from build123d import *

# Parameters (mm, degrees)
SKETCH2_R           = 2.5
BOSS_EXTRUDE1_DEPTH = 3


with BuildPart() as part:
    # Sketch2 → Boss-Extrude1 (new body)
    with BuildSketch(Plane(origin=(0, 0, 0), x_dir=(1, 0, 0), z_dir=(0, 1, 0))):
        with BuildLine():
            Line((-43.63, 60), (43.63, 60))
            ThreePointArc((43.63, 60), (46.896833329, 58.646833329), (48.25, 55.38))
            Line((48.25, 55.38), (48.25, 4.62))
            ThreePointArc((48.25, 4.62), (46.896833329, 1.353166671), (43.63, 0))
            Line((43.63, 0), (-43.63, 0))
            ThreePointArc((-43.63, 0), (-46.896833329, 1.353166671), (-48.25, 4.62))
            Line((-48.25, 4.62), (-48.25, 55.38))
            ThreePointArc((-48.25, 55.38), (-46.896833329, 58.646833329), (-43.63, 60))
        make_face()
        with Locations((-42.13, 6.43)):
            Circle(SKETCH2_R, mode=Mode.SUBTRACT)
        with Locations((-42.13, 53.57)):
            Circle(SKETCH2_R, mode=Mode.SUBTRACT)
        with Locations((5.01, 53.57)):
            Circle(SKETCH2_R, mode=Mode.SUBTRACT)
        with Locations((5.01, 6.43)):
            Circle(SKETCH2_R, mode=Mode.SUBTRACT)
        with BuildLine():
            Line((18.61, 52.5), (40.21, 52.5))
            ThreePointArc((40.21, 52.5), (42.71, 50), (40.21, 47.5))
            Line((40.21, 47.5), (18.61, 47.5))
            ThreePointArc((18.61, 47.5), (16.11, 50), (18.61, 52.5))
        make_face(mode=Mode.SUBTRACT)
        with BuildLine():
            Line((18.61, 7.5), (40.21, 7.5))
            ThreePointArc((40.21, 7.5), (42.71, 10), (40.21, 12.5))
            Line((40.21, 12.5), (18.61, 12.5))
            ThreePointArc((18.61, 12.5), (16.11, 10), (18.61, 7.5))
        make_face(mode=Mode.SUBTRACT)
        with BuildLine():
            Line((18.61, 32.5), (40.21, 32.5))
            ThreePointArc((40.21, 32.5), (42.71, 30), (40.21, 27.5))
            Line((40.21, 27.5), (18.61, 27.5))
            ThreePointArc((18.61, 27.5), (16.11, 30), (18.61, 32.5))
        make_face(mode=Mode.SUBTRACT)
        with BuildLine():
            Line((18.61, 42.5), (40.21, 42.5))
            ThreePointArc((40.21, 42.5), (42.71, 40), (40.21, 37.5))
            Line((40.21, 37.5), (18.61, 37.5))
            ThreePointArc((18.61, 37.5), (16.11, 40), (18.61, 42.5))
        make_face(mode=Mode.SUBTRACT)
        with BuildLine():
            Line((18.61, 17.5), (40.21, 17.5))
            ThreePointArc((40.21, 17.5), (42.71, 20), (40.21, 22.5))
            Line((40.21, 22.5), (18.61, 22.5))
            ThreePointArc((18.61, 22.5), (16.11, 20), (18.61, 17.5))
        make_face(mode=Mode.SUBTRACT)
        with BuildLine():
            Line((-5.025372417, 45.790298215), (-4.191590206, 46.624080426))
            ThreePointArc((-4.191590206, 46.624080426), (-1.935919574, 46.624080426), (-1.935919574, 44.368409794))
            Line((-1.935919574, 44.368409794), (-2.769701785, 43.534627583))
            Line((-2.769701785, 43.534627583), (-2.769701785, 42.274627583))
            ThreePointArc((-2.769701785, 42.274627583), (1.44, 30), (-2.769701785, 17.725372417))
            Line((-2.769701785, 17.725372417), (-2.769701785, 16.465372417))
            Line((-2.769701785, 16.465372417), (-1.935919574, 15.631590206))
            ThreePointArc((-1.935919574, 15.631590206), (-1.935919574, 13.375919574), (-4.191590206, 13.375919574))
            Line((-4.191590206, 13.375919574), (-5.025372417, 14.209701785))
            Line((-5.025372417, 14.209701785), (-6.285372417, 14.209701785))
            ThreePointArc((-6.285372417, 14.209701785), (-18.56, 10), (-30.834627583, 14.209701785))
            Line((-30.834627583, 14.209701785), (-32.094627583, 14.209701785))
            Line((-32.094627583, 14.209701785), (-32.928409794, 13.375919574))
            ThreePointArc((-32.928409794, 13.375919574), (-35.184080426, 13.375919574), (-35.184080426, 15.631590206))
            Line((-35.184080426, 15.631590206), (-34.350298215, 16.465372417))
            Line((-34.350298215, 16.465372417), (-34.350298215, 17.725372417))
            ThreePointArc((-34.350298215, 17.725372417), (-38.56, 30), (-34.350298215, 42.274627583))
            Line((-34.350298215, 42.274627583), (-34.350298215, 43.534627583))
            Line((-34.350298215, 43.534627583), (-35.184080426, 44.368409794))
            ThreePointArc((-35.184080426, 44.368409794), (-35.184080426, 46.624080426), (-32.928409794, 46.624080426))
            Line((-32.928409794, 46.624080426), (-32.094627583, 45.790298215))
            Line((-32.094627583, 45.790298215), (-30.834627583, 45.790298215))
            ThreePointArc((-30.834627583, 45.790298215), (-18.56, 50), (-6.285372417, 45.790298215))
            Line((-6.285372417, 45.790298215), (-5.025372417, 45.790298215))
        make_face(mode=Mode.SUBTRACT)
    extrude(amount=BOSS_EXTRUDE1_DEPTH)


solid = part.part
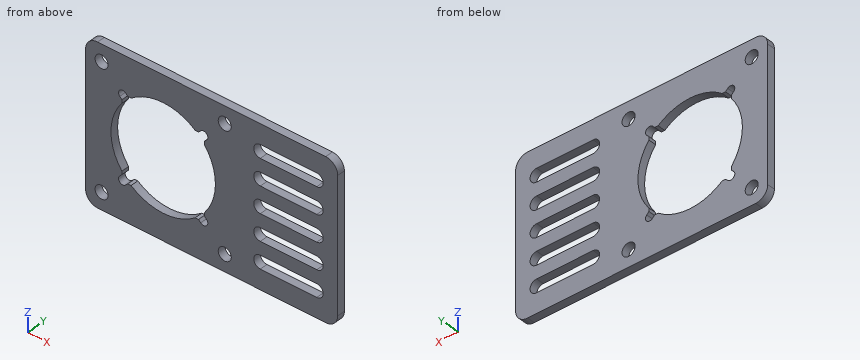
Model file for the job. Use its own axes, mm. Give positions to 0.01 mm unless a question says otherwise; leave off trailing zeros. Order: outer loops, then holes, each group sorted by start corner. A loop starts at its lowest first (then second) coordinate and runs counter-clockwise, first axis right, second up. Notation, with made-up numbers: (-36, -5.5) - (-28, -5.5) arc R30 ccw to (-28, 29.5) - close; hole circle Ø5 at (67.25, 49.5). An arc over 180 degrees is marked (long way). Write item = value, one per line. Start each with the question number.
1. Cut at A-A, the plane z = -30. List the corners of the cut face in (x, y), and give its area (3 significant figures).
2. Cut at C-C, the plane x = 5. List the corners of the cut face in (y, z).
3. Cut at B-B, the plane x = 22.5. List the corners of the cut face in (y, z), and give its area (3 significant figures).
4. Cut at D-D, the plane y = 0.65. State how many separate pieces and enclosed holes the cut face has, and give its area (3 significant figures).
5. Probe line 1 along Z through (x, y) = (-42.13, 1.8); line 2 along X through (y, z) = (0.6, -6.43); line 3 along Z through (x, y) = (-6, 0.8). List the from-to ranges inside material, lowest first.
Taken from the geometry:
q1.outline = (-48.25, 0) - (-38.56, 0) - (-38.56, 3) - (-48.25, 3) - close; (1.44, 0) - (16.11, 0) - (16.11, 3) - (1.44, 3) - close; (42.71, 0) - (48.25, 0) - (48.25, 3) - (42.71, 3) - close
q1.area = 89.7 mm²
q2.outline = (0, -60) - (3, -60) - (3, -56.07) - (0, -56.07) - close; (0, -51.07) - (3, -51.07) - (3, -8.93) - (0, -8.93) - close; (0, -3.93) - (3, -3.93) - (3, 0) - (0, 0) - close
q3.outline = (0, -60) - (3, -60) - (3, -52.5) - (0, -52.5) - close; (0, -47.5) - (3, -47.5) - (3, -42.5) - (0, -42.5) - close; (0, -37.5) - (3, -37.5) - (3, -32.5) - (0, -32.5) - close; (0, -27.5) - (3, -27.5) - (3, -22.5) - (0, -22.5) - close; (0, -17.5) - (3, -17.5) - (3, -12.5) - (0, -12.5) - close; (0, -7.5) - (3, -7.5) - (3, 0) - (0, 0) - close
q3.area = 105 mm²
q4.separate_pieces = 1
q4.enclosed_holes = 10
q4.area = 3,750 mm²
q5.line_1 = -60 to -56.07, -51.07 to -8.93, -3.93 to 0
q5.line_2 = -48.25 to -44.63, -39.63 to 2.51, 7.51 to 48.25
q5.line_3 = -60 to -45.79, -14.21 to 0
